The listing builds one solid part. Answer for the finished solid, in the listing's coordinates (mm). Face numbers are marked on the shaded views. A direction names the side the tool comes from. Coordinates: 2 decimals unless noted, no trailing zeros. Order: outer loops, then holes, each group sorted by start corner. A loop starts at its lowest first (then second) coordinate and runs counter-clockwise, first axis right, second up. Notation, with made-up numbers: (65, -8.5) -> (101, -8.5) arc R18 ccw to (101, 26.5) -> close; hole circle Ø6 at (61, 69.25). An arc over 180 degrees is marked (long way). Return JSON: item names as keys, results as strings.
```python
from build123d import *

# Parameters (mm, degrees)
SKETCH1_R           = 132
BOSS_EXTRUDE1_DEPTH = 5
SKETCH2_R           = 132
SKETCH2_R_2         = 125
BOSS_EXTRUDE2_DEPTH = 90
SKETCH3_W           = 49.925821921
SKETCH3_H           = 40
BOSS_EXTRUDE4_DEPTH = 50
SKETCH4_W           = 40.744064535
SKETCH4_H           = 32
CUT_EXTRUDE1_DEPTH  = 40
SKETCH5_R           = 8
CUT_EXTRUDE2_DEPTH  = 40
CIRPATTERN2_COUNT   = 4
SKETCH7_R           = 32
SKETCH7_R_2         = 28
CUT_EXTRUDE3_DEPTH  = 2
SKETCH8_R           = 6
CUT_EXTRUDE4_DEPTH  = 3
BOSS_EXTRUDE5_START = -5
SKETCH9_R           = 32
BOSS_EXTRUDE5_DEPTH = 5
SKETCH10_R          = 32
SKETCH10_R_2        = 24
CUT_EXTRUDE5_DEPTH  = 2
SKETCH11_R          = 14
SKETCH11_R_2        = 6
CUT_EXTRUDE6_DEPTH  = 2
SKETCH12_R          = 6
CUT_EXTRUDE7_DEPTH  = 3


with BuildPart() as part:
    # Sketch1 → Boss-Extrude1 (new body)
    with BuildSketch(Plane(origin=(0, 0, 0), x_dir=(1, 0, 0), z_dir=(0, 1, 0))):
        with Locations(Location((0, 0, 0), (0, 0, 270))):
            Circle(SKETCH1_R)
    extrude(amount=BOSS_EXTRUDE1_DEPTH)

    # Sketch2 → Boss-Extrude2 (add)
    with BuildSketch(Plane(origin=(0, 5, 0), x_dir=(1, 0, 0), z_dir=(0, 1, 0))):
        with Locations(Location((0, 0, 0), (0, 0, 270))):
            Circle(SKETCH2_R)
        with Locations(Location((0, 0, 0), (0, 0, 270))):
            Circle(SKETCH2_R_2, mode=Mode.SUBTRACT)
    extrude(amount=BOSS_EXTRUDE2_DEPTH)

    # Sketch3 → Boss-Extrude4 (add)
    with BuildSketch(Plane.XZ):
        with Locations((-152.03708904, 0)):
            Rectangle(SKETCH3_W, SKETCH3_H)
    extrude(amount=-BOSS_EXTRUDE4_DEPTH)

    # Sketch4 → Cut-Extrude1 (cut)
    with BuildSketch(Plane(origin=(0, 50, 0), x_dir=(1, 0, 0), z_dir=(0, 1, 0))):
        with Locations((-156.627967732, 0)):
            Rectangle(SKETCH4_W, SKETCH4_H)
    extrude(amount=-CUT_EXTRUDE1_DEPTH, mode=Mode.SUBTRACT)

    # Sketch5 → Cut-Extrude2 (cut)
    with BuildSketch(Plane(origin=(0, 10, 0), x_dir=(1, 0, 0), z_dir=(0, 1, 0))):
        with Locations(Location((-157.186334462, 0, 0), (0, 0, 270))):
            Circle(SKETCH5_R)
    extrude(amount=-CUT_EXTRUDE2_DEPTH, mode=Mode.SUBTRACT)


with BuildPart() as cirpattern2_1:
    # CirPattern2: pattern copy
    add(part.part.rotate(Axis((0, 0, 0), (0, 1, 0)), 1 * 360 / CIRPATTERN2_COUNT))


with BuildPart() as cirpattern2_2:
    # CirPattern2: pattern copy
    add(part.part.rotate(Axis((0, 0, 0), (0, 1, 0)), 2 * 360 / CIRPATTERN2_COUNT))


with BuildPart() as cirpattern2_3:
    # CirPattern2: pattern copy
    add(part.part.rotate(Axis((0, 0, 0), (0, 1, 0)), 3 * 360 / CIRPATTERN2_COUNT))


with BuildPart() as cut_extrude3_tool:
    # Sketch7 → Cut-Extrude3 (new body)
    with BuildSketch(Plane(origin=(0, 5, 0), x_dir=(1, 0, 0), z_dir=(0, 1, 0))):
        with Locations(Location((0, 0, 0), (0, 0, 270))):
            Circle(SKETCH7_R)
        with Locations(Location((0, 0, 0), (0, 0, 270))):
            Circle(SKETCH7_R_2, mode=Mode.SUBTRACT)
    extrude(amount=-CUT_EXTRUDE3_DEPTH)


with BuildPart() as part_1:
    add(part.part)

    # Cut-Extrude3: cut by cut_extrude3_tool
    add(cut_extrude3_tool.part, mode=Mode.SUBTRACT)


with BuildPart() as cirpattern2_1_1:
    add(cirpattern2_1.part)

    # Cut-Extrude3: cut by cut_extrude3_tool
    add(cut_extrude3_tool.part, mode=Mode.SUBTRACT)


with BuildPart() as cirpattern2_2_1:
    add(cirpattern2_2.part)

    # Cut-Extrude3: cut by cut_extrude3_tool
    add(cut_extrude3_tool.part, mode=Mode.SUBTRACT)


with BuildPart() as cirpattern2_3_1:
    add(cirpattern2_3.part)

    # Cut-Extrude3: cut by cut_extrude3_tool
    add(cut_extrude3_tool.part, mode=Mode.SUBTRACT)


with BuildPart() as cut_extrude4_tool:
    # Sketch8 → Cut-Extrude4 (new body)
    with BuildSketch(Plane(origin=(0, 5, 0), x_dir=(1, 0, 0), z_dir=(0, 1, 0))):
        with Locations(Location((0, 0, 0), (0, 0, 270))):
            Circle(SKETCH8_R)
    extrude(amount=-CUT_EXTRUDE4_DEPTH)


with BuildPart() as part_2:
    add(part_1.part)

    # Cut-Extrude4: cut by cut_extrude4_tool
    add(cut_extrude4_tool.part, mode=Mode.SUBTRACT)



with BuildPart() as cirpattern2_1_2:
    add(cirpattern2_1_1.part)

    # Cut-Extrude4: cut by cut_extrude4_tool
    add(cut_extrude4_tool.part, mode=Mode.SUBTRACT)


with BuildPart() as cirpattern2_2_2:
    add(cirpattern2_2_1.part)

    # Cut-Extrude4: cut by cut_extrude4_tool
    add(cut_extrude4_tool.part, mode=Mode.SUBTRACT)


with BuildPart() as cirpattern2_3_2:
    add(cirpattern2_3_1.part)

    # Cut-Extrude4: cut by cut_extrude4_tool
    add(cut_extrude4_tool.part, mode=Mode.SUBTRACT)


with BuildPart() as part_3:
    add(part_2.part)

    add(cirpattern2_1_2.part)  # Boss-Extrude5 merges CirPattern2_1

    add(cirpattern2_2_2.part)  # Boss-Extrude5 merges CirPattern2_2

    add(cirpattern2_3_2.part)  # Boss-Extrude5 merges CirPattern2_3
    # Sketch9 → Boss-Extrude5 (add)
    with BuildSketch(Plane.XZ.offset(BOSS_EXTRUDE5_START)):
        Circle(SKETCH9_R)
    extrude(amount=BOSS_EXTRUDE5_DEPTH)

    # Sketch10 → Cut-Extrude5 (cut)
    with BuildSketch(Plane(origin=(0, 5, 0), x_dir=(1, 0, 0), z_dir=(0, 1, 0))):
        with Locations(Location((0, 0, 0), (0, 0, 270))):
            Circle(SKETCH10_R)
        with Locations(Location((0, 0, 0), (0, 0, 270))):
            Circle(SKETCH10_R_2, mode=Mode.SUBTRACT)
    extrude(amount=-CUT_EXTRUDE5_DEPTH, mode=Mode.SUBTRACT)

    # Sketch11 → Cut-Extrude6 (cut)
    with BuildSketch(Plane(origin=(0, 5, 0), x_dir=(1, 0, 0), z_dir=(0, 1, 0))):
        with Locations(Location((0, 0, 0), (0, 0, 270))):
            Circle(SKETCH11_R)
        with Locations(Location((0, 0, 0), (0, 0, 270))):
            Circle(SKETCH11_R_2, mode=Mode.SUBTRACT)
    extrude(amount=-CUT_EXTRUDE6_DEPTH, mode=Mode.SUBTRACT)

    # Sketch12 → Cut-Extrude7 (cut)
    with BuildSketch(Plane(origin=(0, 5, 0), x_dir=(1, 0, 0), z_dir=(0, 1, 0))):
        with Locations(Location((0, 0, 0), (0, 0, 270))):
            Circle(SKETCH12_R)
    extrude(amount=-CUT_EXTRUDE7_DEPTH, mode=Mode.SUBTRACT)


solid = part_3.part
```
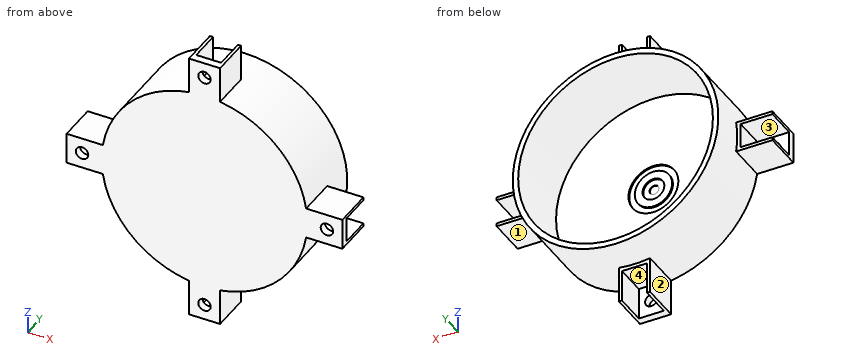
Item 1: The part is cut by section B-B on y = 87. Determine the outline of the cut face in (x, z), plus the area to 3 significant figures.
Answer list:
{"outline": "circle Ø264 at (0, 0); hole circle Ø250 at (0, 0)", "area": "5,650 mm2"}
Item 2: Which of the six approach directions +Z, -Z, +X, -X, +Y, -Y give full straight-line access (tool end or side, diameter ignored) to the marked faces 1, 2, 3 and 4?
Answer list:
{"face 1": "-Z, +X, +Y, -Y", "face 2": "-Z, -X, +Y, -Y", "face 3": "-X, +Y", "face 4": "-Z, +Y"}
Item 3: The part is cut by section A-A on x = 0. Count the separate pieces of the cut face and the enclosed holes in it, plus the area to 3 significant figures.
Answer list:
{"separate pieces": "3", "enclosed holes": "0", "area": "3,400 mm2"}
Item 4: The part is cut by section D-D on z = -56. Determine the outline of the cut face in (x, y), plus the area to 3 significant figures.
Answer list:
{"outline": "(-119.53, 0) -> (119.53, 0) -> (119.53, 95) -> (111.75, 95) -> (111.75, 5) -> (-111.75, 5) -> (-111.75, 95) -> (-119.53, 95) -> close", "area": "2,600 mm2"}
Item 5: Find the intervals of material crossed by probe 1 along Z at (x, y) = (0, 34); probe 2 along Y at (x, z) = (51.5, -55.5); probe 3 along X at (y, z) = (65, 115.5), in increasing order.
Answer list:
{"probe 1": "-136.26 to -125, 125 to 136.26", "probe 2": "0 to 5", "probe 3": "-63.9 to -47.8, 47.8 to 63.9"}
Item 6: Flat-ended cylindrical pins translate along their axes: pin 1 (12 mm diameter, centred on x = -105.5, y = 24, fed in from -Z); pin 2 (20 mm diameter, centred on x = 9, z = -161, fed in from +Y); pin 3 (13 mm diameter, centred on x = 1.5, z = -1, fed in from +Y); pin 4 (9.5 mm diameter, centred on x = 0, z = 157.19, fed in from -Y). Find the tip coordinate at first contact, or state that the pin passes through.
Answer list:
{"pin 1": "z = -86.74", "pin 2": "y = 50", "pin 3": "y = 3", "pin 4": "through"}
